Print and shaded views of the part. All mm, measured from the part's lowest x, y and z. Coordinates: 2 decimals unless noted, no trailing zeros. Write each loop counter-clockwise with the first axis right and the second up, starting at its lowest first coordinate (ties: lowest second). Pieces come first, ordered by that corner, then holes. Notation, with made-up numbers: (-32, -6.5) -> (0, -6.5) arc R22 cw to (0, 12.5) -> close; hole circle Ø9 at (17.5, -11.5). An arc over 180 degrees is marked (long way). Write item = value, one per line.
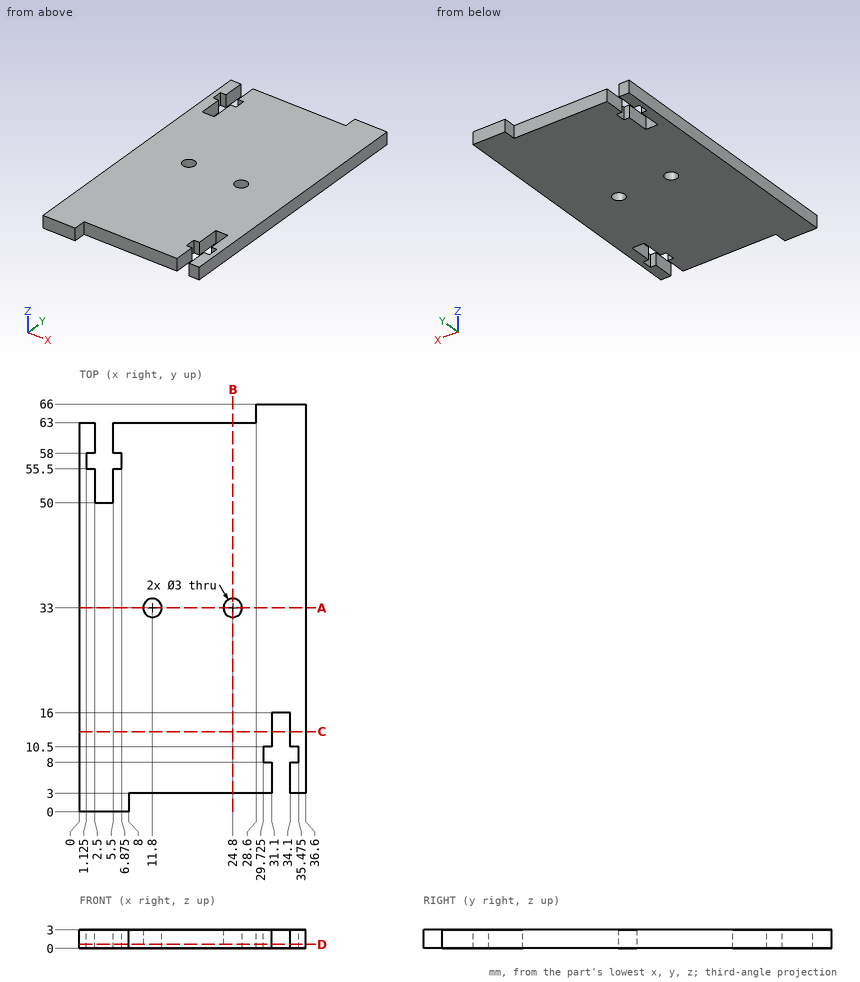
Q1. Saw through at C-C on y = 13. Give the cut face in (x, z), and give its area (3 significant figures).
Model answer:
outline = (0, 0) -> (31.1, 0) -> (31.1, 3) -> (0, 3) -> close; (34.1, 0) -> (36.6, 0) -> (36.6, 3) -> (34.1, 3) -> close
area = 101 mm²
Q2. Saw through at A-A on y = 33. Give the cut face in (x, z), and give its area (3 significant figures).
Model answer:
outline = (0, 0) -> (10.3, 0) -> (10.3, 3) -> (0, 3) -> close; (13.3, 0) -> (23.3, 0) -> (23.3, 3) -> (13.3, 3) -> close; (26.3, 0) -> (36.6, 0) -> (36.6, 3) -> (26.3, 3) -> close
area = 91.8 mm²
Q3. Saw through at D-D on z = 0.65. Count the separate pieces of the cut face and the enclosed holes in it, and give its area (3 significant figures).
Model answer:
separate_pieces = 1
enclosed_holes = 2
area = 2,140 mm²
Q4. Saw through at B-B on x = 24.8. Give the cut face in (y, z).
Model answer:
outline = (3, 0) -> (31.5, 0) -> (31.5, 3) -> (3, 3) -> close; (34.5, 0) -> (63, 0) -> (63, 3) -> (34.5, 3) -> close
Q5. Pin check, flat tips, straight feed: pin 1 (1.5 mm diameter, centred on y = 65, z = 2, fed in from -X); pin 2 (1.5 mm diameter, centred on x = 34.5, z = 2, fed in from -Y); pin 3 (1.5 mm diameter, centred on x = 18.5, z = 2.5, fed in from +Y); pin 4 (0.9 mm diameter, centred on y = 5, z = 1.5, fed in from -X). Stop position of each tip, or through.
Model answer:
pin_1 = 28.6
pin_2 = 3
pin_3 = 63
pin_4 = 0
Q6. Probe line 1 (Y direction, x = 6, z = 1.65); line 2 (Y direction, x = 11.8, z = 1.25); line 3 (X direction, y = 6, z = 1.2). List the from-to ranges inside material, lowest first. Write a range as from..to.
Model answer:
line_1 = 0..55.5, 58..63
line_2 = 3..31.5, 34.5..63
line_3 = 0..31.1, 34.1..36.6
